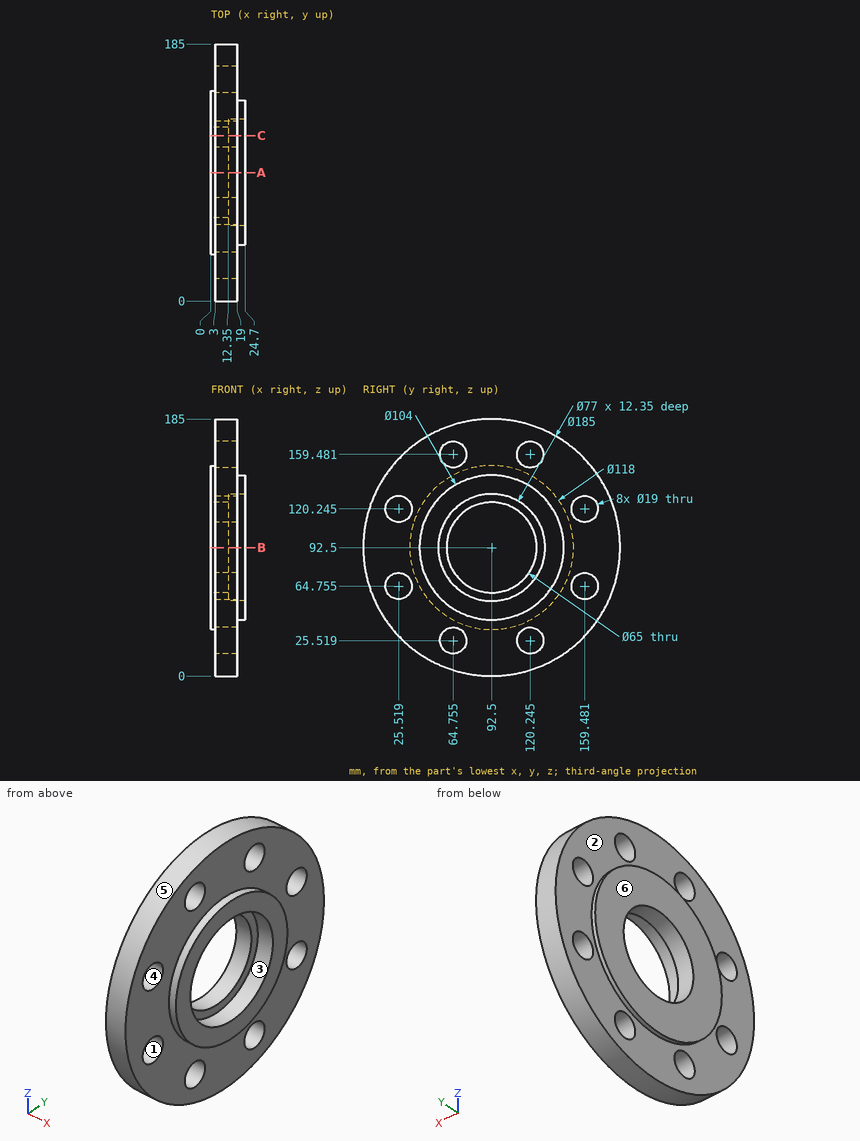
The drawing under review shows one solid part. Ordinate dimensions are in mm from its lowest x, y, z. A direction names the side the tool comes from. Coordinates: 2 decimals unless noted, no trailing zeros. Order: outer loops, then holes, each group sorted by start corner. A loop starts at its lowest first (then second) coordinate and runs counter-clockwise, first axis right, second up. Notation, with made-up numbers: M 7,33.25 L 60,33.25 A27 cw 60,68.25 Z; hole C 85.5,-8.5 d9. An arc over 180 degrees is marked long. Use a Markdown table: item, result.
(1) Draft analysis for pull direction Y (two halves, no side actions). For the marked faces 4, 5 and 6, state which applies: released by +Y, released by -Y, zero draft, split by the parting line, or undercut.
Worked answers:
| item | result |
|---|---|
| face 4 | undercut |
| face 5 | split by the parting line |
| face 6 | zero draft |
(2) Wall thickness on probe 1 along Z at (x, y) = (21, 92.5); probe 2 along Z at (x, y) = (16, 73.5) (1 decimal); probe 3 along Z at (x, y) = (7.25, 128.5) (1 decimal): over which ranges is each line inside the solid? List them lowest first.
Worked answers:
| item | result |
|---|---|
| probe 1 | z = 40.5 to 54, 131 to 144.5 |
| probe 2 | z = 2 to 21.8, 29.2 to 59, 126 to 155.8, 163.2 to 183 |
| probe 3 | z = 7.3 to 20.8, 30.2 to 154.8, 164.2 to 177.7 |
(3) Add section C-C (y = 119). Count the separate pieces of the cut face and the enclosed holes in it, then the cut area to 4 significant figures.
Worked answers:
| item | result |
|---|---|
| separate pieces | 4 |
| enclosed holes | 0 |
| area | 1,905 mm2 |
(4) For the marked faces 1, 2 and 3, list the 3-axis set-ups (+Z, -Z, +X, -X, +Y, -Y) from which the entire face can be reached by the end or side of a thin tool; tool diameter is ignored.
Worked answers:
| item | result |
|---|---|
| face 1 | +X, -X |
| face 2 | -X |
| face 3 | +X |
(5) For P1, Ø8, axis at x = 13.5, z = 78.5, coming from the -Y side; P2, Ø3, axis at y = 151, z = 160.5, coming from the -X side; P3, Ø15, axis at y = 25.52, z = 120.24, coming from the +X side; P4, Ø24.5, axis at y = 64.76, z = 25.52, coming from the +X side, all flat-tipped, find the tip position at first contact; note any pin that passes through.
Worked answers:
| item | result |
|---|---|
| P1 | stops at y = 0.54 |
| P2 | stops at x = 3 |
| P3 | passes through |
| P4 | stops at x = 19 |
(6) Add section A-A (y = 92.5). Give the boundary of the cut face in (x, z), then the cut area to 3 significant figures.
Worked answers:
| item | result |
|---|---|
| outline | M 0,33.5 L 3,33.5 L 3,0 L 19,0 L 19,40.5 L 24.7,40.5 L 24.7,54 L 12.35,54 L 12.35,60 L 0,60 Z; M 0,125 L 12.35,125 L 12.35,131 L 24.7,131 L 24.7,144.5 L 19,144.5 L 19,185 L 3,185 L 3,151.5 L 0,151.5 Z |
| area | 2,150 mm2 |
